from build123d import *

# Parameters (mm, degrees)
SKETCH1_W                 = 762
SKETCH1_H                 = 69.85
BOSS_EXTRUDE1_DEPTH       = 9.525
HOLE1_D                   = 6
HOLE1_CBORE_D             = 12
HOLE1_CBORE_DEPTH         = 4.1
M4X0_7_TAPPED_HOLE1_D     = 3.3
M4X0_7_TAPPED_HOLE1_DEPTH = 10.1
M4X0_7_TAPPED_HOLE1_TIP   = 0.991420021
M5X0_8_TAPPED_HOLE1_D     = 4.2
M5X0_8_TAPPED_HOLE1_DEPTH = 12.4
M5X0_8_TAPPED_HOLE1_TIP   = 1.2618073


with BuildPart() as part:
    # Sketch1 → Boss-Extrude1 (new body)
    with BuildSketch(Plane.XY):
        with Locations((381, 34.925)):
            Rectangle(SKETCH1_W, SKETCH1_H)
    extrude(amount=BOSS_EXTRUDE1_DEPTH)

    # Hole1 (through all)
    with Locations(Plane(origin=(750, 59.925, 0), x_dir=(-1, 0, 0), z_dir=(0, 0, -1))):
        with Locations((0, 0), (0, -50), (369, 0), (369, -50), (738, 0), (738, -50)):
            CounterBoreHole(HOLE1_D / 2, HOLE1_CBORE_D / 2, HOLE1_CBORE_DEPTH)

    # M4x0.7 Tapped Hole1
    with Locations(Plane(origin=(741, 34.925, 0), x_dir=(-1, 0, 0), z_dir=(0, 0, -1))):
        with Locations((0, 0), (60, 0), (120, 0), (180, 0), (240, 0), (300, 0), (360, 0), (420, 0), (480, 0), (540, 0), (600, 0), (660, 0), (720, 0)):
            Hole(M4X0_7_TAPPED_HOLE1_D / 2, depth=M4X0_7_TAPPED_HOLE1_DEPTH)
            with Locations((0, 0, -(M4X0_7_TAPPED_HOLE1_DEPTH + M4X0_7_TAPPED_HOLE1_TIP / 2))):  # 118° drill point
                Cone(0, M4X0_7_TAPPED_HOLE1_D / 2, M4X0_7_TAPPED_HOLE1_TIP, mode=Mode.SUBTRACT)

    # M5x0.8 Tapped Hole1
    with Locations(Plane(origin=(629, 49.925, 0), x_dir=(-1, 0, 0), z_dir=(0, 0, -1))):
        with Locations((0, 0), (0, -30), (100, 0), (100, -30), (200, 0), (200, -30), (300, 0), (300, -30), (400, 0), (400, -30), (500, 0), (500, -30)):
            Hole(M5X0_8_TAPPED_HOLE1_D / 2, depth=M5X0_8_TAPPED_HOLE1_DEPTH)
            with Locations((0, 0, -(M5X0_8_TAPPED_HOLE1_DEPTH + M5X0_8_TAPPED_HOLE1_TIP / 2))):  # 118° drill point
                Cone(0, M5X0_8_TAPPED_HOLE1_D / 2, M5X0_8_TAPPED_HOLE1_TIP, mode=Mode.SUBTRACT)


solid = part.part
Geometry check sheet. Reference: the model listing, model coordinates, mm. A direction names the side the tool comes from. Round coordinates to 2 decimals unless told otherwise and drop trailing zeros. One line per question, with ' | ' between items. Start each with the question number.
(1) Depth check by flat-ended pin: pin 1 Ø4 at (x, y) = (129, 19.925) entering from -Z; pin 2 Ø6 at (x, y) = (750, 11.5) entering from -Z. Enter the tip coordinate at first touch or a pass-through.
(2) Access from +Z, -Z, +X, -X, +Y, -Y to the whole of each face (thin tool, end or side, straight path). Record for faces 4 (the cylindrical face through (377.8, 15, 2)), 5 (the flat face through (376, 35, 0)).
(3) Thickness scan on L1, parallel to Y at x = 529, z = 6.5 (3 decimals); L2, parallel to Y at x = 12, z = 0.9 (3 decimals); L3, parallel to X at y = 63, z = 0.5. Record the ranges inside material, lowest first. Write a range as [from, to].
(4) Release check for a two-part mould opening along Y. For faces 1 (the flat face through (376, 35, 9.525)), 2 (the flat face through (11, 13, 4.1)), 3 (the cylindrical face through (8.8, 65, 2)) record: released by +Y, released by -Y, zero draft, split by the parting line, or undercut.
Conclusion:
1) pin 1: passes through | pin 2: stops at z = 4.1
2) face 4: -Z | face 5: -Z, +X, -X, +Y, -Y
3) L1: y = [0, 17.825], [22.025, 47.825], [52.025, 69.85] | L2: y = [0, 3.925], [15.925, 53.925], [65.925, 69.85] | L3: x = [0, 6.85], [17.15, 375.85], [386.15, 744.85], [755.15, 762]
4) face 1: zero draft | face 2: undercut | face 3: undercut
